```python
from build123d import *

# Parameters (mm, degrees)
F0_R     = 47.2948
F1_DEPTH = 19.05


with BuildPart() as f1:
    # F0 (on Top) → F1 (new body)
    with BuildSketch(Plane.XY):
        Circle(F0_R)
        with BuildLine():
            ThreePointArc((42.505515, 2.3495), (42.554176, 1.175198), (42.5704, 0))
            ThreePointArc((42.5704, 0), (42.554176, -1.175198), (42.505515, -2.3495))
            ThreePointArc((42.505515, -2.3495), (30.101819, -30.101819), (2.3495, -42.505515))
            ThreePointArc((2.3495, -42.505515), (0, -42.5704), (-2.3495, -42.505515))
            ThreePointArc((-2.3495, -42.505515), (-30.101819, -30.101819), (-42.505515, -2.3495))
            ThreePointArc((-42.505515, -2.3495), (-42.5704, 0), (-42.505515, 2.3495))
            ThreePointArc((-42.505515, 2.3495), (-30.101819, 30.101819), (-2.3495, 42.505515))
            ThreePointArc((-2.3495, 42.505515), (0, 42.5704), (2.3495, 42.505515))
            ThreePointArc((2.3495, 42.505515), (30.101819, 30.101819), (42.505515, 2.3495))
        make_face(mode=Mode.SUBTRACT)
        with BuildLine():
            Line((2.3495, 9.584117), (2.3495, 42.505515))
            ThreePointArc((2.3495, 42.505515), (0, 42.5704), (-2.3495, 42.505515))
            Line((-2.3495, 42.505515), (-2.3495, 9.584117))
            ThreePointArc((-2.3495, 9.584117), (0, 9.8679), (2.3495, 9.584117))
        make_face()
        with BuildLine():
            ThreePointArc((9.8679, 0), (9.796697, 1.183288), (9.584117, 2.3495))
            ThreePointArc((9.584117, 2.3495), (6.977659, 6.977659), (2.3495, 9.584117))
            ThreePointArc((2.3495, 9.584117), (0, 9.8679), (-2.3495, 9.584117))
            ThreePointArc((-2.3495, 9.584117), (-6.977659, 6.977659), (-9.584117, 2.3495))
            ThreePointArc((-9.584117, 2.3495), (-9.8679, 0), (-9.584117, -2.3495))
            ThreePointArc((-9.584117, -2.3495), (-6.977659, -6.977659), (-2.3495, -9.584117))
            ThreePointArc((-2.3495, -9.584117), (0, -9.8679), (2.3495, -9.584117))
            ThreePointArc((2.3495, -9.584117), (6.977659, -6.977659), (9.584117, -2.3495))
            ThreePointArc((9.584117, -2.3495), (9.796697, -1.183288), (9.8679, 0))
        make_face()
        Polygon((-5.207, 3.006263), (0, 6.012526), (5.207, 3.006263), (5.207, -3.006263), (0, -6.012526), (-5.207, -3.006263), align=None, mode=Mode.SUBTRACT)
        with BuildLine():
            Line((-9.584117, 2.3495), (-42.505515, 2.3495))
            ThreePointArc((-42.505515, 2.3495), (-42.5704, 0), (-42.505515, -2.3495))
            Line((-42.505515, -2.3495), (-9.584117, -2.3495))
            ThreePointArc((-9.584117, -2.3495), (-9.8679, 0), (-9.584117, 2.3495))
        make_face()
        with BuildLine():
            ThreePointArc((-2.3495, -42.505515), (0, -42.5704), (2.3495, -42.505515))
            Line((2.3495, -42.505515), (2.3495, -9.584117))
            ThreePointArc((2.3495, -9.584117), (0, -9.8679), (-2.3495, -9.584117))
            Line((-2.3495, -9.584117), (-2.3495, -42.505515))
        make_face()
        with BuildLine():
            ThreePointArc((42.505515, -2.3495), (42.554176, -1.175198), (42.5704, 0))
            ThreePointArc((42.5704, 0), (42.554176, 1.175198), (42.505515, 2.3495))
            Line((42.505515, 2.3495), (9.584117, 2.3495))
            ThreePointArc((9.584117, 2.3495), (9.796697, 1.183288), (9.8679, 0))
            ThreePointArc((9.8679, 0), (9.796697, -1.183288), (9.584117, -2.3495))
            Line((9.584117, -2.3495), (42.505515, -2.3495))
        make_face()
    extrude(amount=F1_DEPTH)


solid = f1.part
```
Could you check a few things on this model? Use its own coordinates, in mm. Round coordinates to 2 decimals unless told otherwise and drop trailing zeros. Loops run counter-clockwise (first coordinate to the right, second up) from the corner with the lowest first, then second, coordinate; pieces in that order, holes last. Notation, with made-up numbers: (6.5, -8.5) -> (57.5, -8.5) arc R20 ccw to (57.5, 4.5) -> close; hole circle Ø1 at (48.5, -14.5). An arc over 180 degrees is marked (long way). Put each result on its own line as item: value.
Q1. I want a section at A-A on z = 7.75. Write out the boundary of the cut face in (x, y).
Checks:
outline: circle Ø94.59 at (0, 0); hole (-42.51, -2.35) arc R42.57 ccw to (-2.35, -42.51) -> (-2.35, -9.58) arc R9.87 cw to (-9.58, -2.35) -> close; hole (-42.51, 2.35) -> (-9.58, 2.35) arc R9.87 cw to (-2.35, 9.58) -> (-2.35, 42.51) arc R42.57 ccw to start; hole (-5.21, -3.01) -> (0, -6.01) -> (5.21, -3.01) -> (5.21, 3.01) -> (0, 6.01) -> (-5.21, 3.01) -> close; hole (2.35, -42.51) arc R42.57 ccw to (42.51, -2.35) -> (9.58, -2.35) arc R9.87 cw to (2.35, -9.58) -> close; hole (2.35, 9.58) arc R9.87 cw to (9.58, 2.35) -> (42.51, 2.35) arc R42.57 ccw to (2.35, 42.51) -> close
Q2. Please list where these lines run through material, in increasing order: line 1 (Y direction, x = -31, z = 2.25); line 2 (Y direction, x = 33, z = 16.25); line 3 (X direction, y = -3, z = 6.75). Write a range as from..to.
Checks:
line 1: -35.72..-29.18, -2.35..2.35, 29.18..35.72
line 2: -33.88..-26.89, -2.35..2.35, 26.89..33.88
line 3: -47.2..-42.46, -9.4..-5.21, 5.21..9.4, 42.46..47.2
Q3. For pin 1 Ø1.5 at (x, z) = (15, 15) entering from +Y; pin 2 Ø5.5 at (y, z) = (32, 6) entering from -X (3 decimals); pin 3 Ø1.5 at (x, z) = (8, 3.5) entering from +Y, each with a flat end and sliding along its axis, tell me the tip position at first contact or that it passes through.
Checks:
pin 1: y = 45.1
pin 2: x = -37.165
pin 3: y = 46.74
Q4. I want a section at B-B on y = -37. Write out the boundary of the cut face in (x, z), and give its area (3 significant figures).
Checks:
outline: (-29.46, 0) -> (-21.05, 0) -> (-21.05, 19.05) -> (-29.46, 19.05) -> close; (-2.35, 0) -> (2.35, 0) -> (2.35, 19.05) -> (-2.35, 19.05) -> close; (21.05, 0) -> (29.46, 0) -> (29.46, 19.05) -> (21.05, 19.05) -> close
area: 410 mm2
Q5. I want a section at D-D on y = 0. Write out the boundary of the cut face in (x, z).
Checks:
outline: (-47.29, 0) -> (-5.21, 0) -> (-5.21, 19.05) -> (-47.29, 19.05) -> close; (5.21, 0) -> (47.29, 0) -> (47.29, 19.05) -> (5.21, 19.05) -> close
Q6. Thinking about a two-plate mould opening in X: for faces 1 (the flat face through (10, 1, 0)), 2 (the cylindrical face through (-6.924, 7.031, 9.392)), 3 (the cylindrical face through (-10.25, -46.17, 9.39)), which applies, pulls with the +X half, pulls with the -X half, needs draft (parallel to the pull), parting line crosses it, or undercut?
Checks:
face 1: needs draft
face 2: undercut
face 3: parting line crosses it
Q7. I want a section at C-C on x = -15.5. Write out the boundary of the cut face in (y, z), and give its area (3 significant figures).
Checks:
outline: (-44.68, 0) -> (-39.65, 0) -> (-39.65, 19.05) -> (-44.68, 19.05) -> close; (-2.35, 0) -> (2.35, 0) -> (2.35, 19.05) -> (-2.35, 19.05) -> close; (39.65, 0) -> (44.68, 0) -> (44.68, 19.05) -> (39.65, 19.05) -> close
area: 281 mm2
